Here's the drawing with two shaded views (mm, measured from the low corner). I have some questions. Give positions to 0.01 mm unless a question says otherwise; leave off trailing zeros. Loops run counter-clockwise (first coordinate to the right, second up) from the corner with the lowest first, then second, coordinate; pieces in that order, holes last. Notation, with made-up numbers: (29.5, -40) - (64.5, -40) arc R18 cw to (64.5, -12) - close; hole circle Ø3 at (15.25, 18.25). An arc over 180 degrees is marked (long way). Use one line per item in the form item = value.
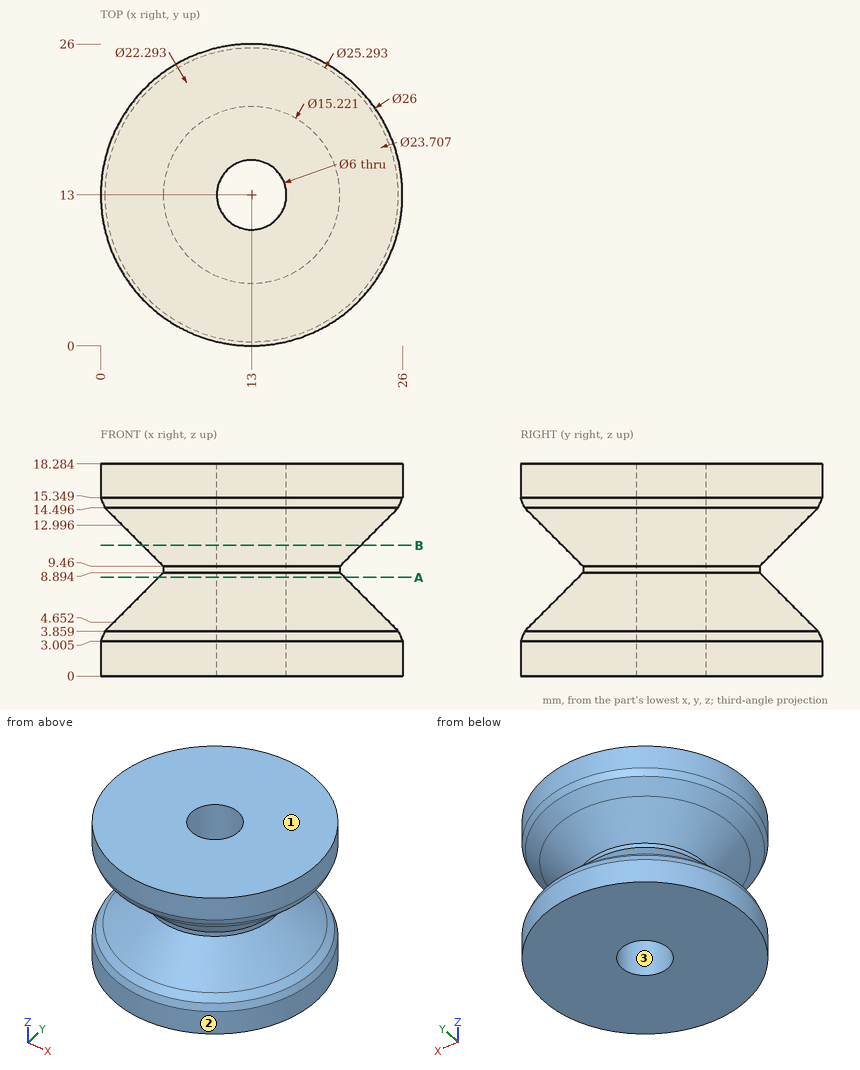
(1) For P1, Ø9.5, axis at x = 13, y = 13, coming from the +Z side; P2, Ø1, axis at x = 21.5, z = 4.5, coming from the +Y side; P3, Ø10, axis at x = 5.5, z = 16, coming from the -Y side; P4, Ø5, axis at x = 21, z = 9.5, coming from the -Y side, each with a flat end and sliding along its axis, tell me the tip position at first contact or that it passes through.
Geometry says:
P1 = 18.28
P2 = 22.31
P3 = 0.24
P4 = 5.86
(2) Thinking about a two-plate mould opening in Y: for the marked faces 1, 2 and 3, which applies, pulls with the +Y half, pulls with the -Y half, needs draft (parallel to the pull), parting line crosses it, or undercut?
Geometry says:
face_1 = needs draft
face_2 = parting line crosses it
face_3 = undercut
(3) If we section it at B-B (z = 11.25): List the corners of the cut face in (x, y) for me.
Geometry says:
outline = circle Ø18.8 at (13, 13); hole circle Ø6 at (13, 13)
(4) If we section it at A-A (z = 8.5): List the corners of the cut face in (x, y) for me (1 decimal).
Geometry says:
outline = circle Ø16 at (13, 13); hole circle Ø6 at (13, 13)
(5) If I drill on probe 1 along X at (y, z) = (13, 8.25) (1 decimal); probe 2 along Y at (x, z) = (13, 13); probe 3 along Z at (x, y) = (21.25, 15) (1 decimal), over which ranges is the centre line in solid material (lowest first)?
Geometry says:
probe_1 = 4.7 to 10, 16 to 21.3
probe_2 = 1.85 to 10, 16 to 24.15
probe_3 = 0 to 8, 10.3 to 18.3
